Could you check a few things on this model? Use its own coordinates, in mm. A direction names the side the tool comes from. Coordinates: 2 decimals unless noted, no trailing zeros. Write each loop counter-clockwise with the first axis right and the second up, starting at its lowest first coordinate (ties: lowest second). Pieces come first, ordered by that corner, then holes. Notation, with made-up numbers: M -27,-25 L -2,-25 A4 ccw -2,-19 Z; hole C -21,49 d3. An arc over 180 degrees is marked long. Answer as CSV lines item,"result". Start each with the question number.
Item 1: Suppose I cut it at A-A, the plane x = -6. Write out the boundary of the cut face in (y, z), and give its area (3 significant figures).
Item 2: On a 3-axis mill with a long thin cutter (end or side, diameter ignored), from which of +Z, -Z, +X, -X, +Y, -Y can I reach the whole of each face in a straight line? I mean faces 3 (the cylindrical face through (35.965, 0.105, -27.525)), 4 (the flat face through (27.8, -2.5, -8)). Say none if no direction works.
Item 3: Suppose I cut it at C-C, the plane y = -1.25. Write out the boundary of the cut face in (x, z), and give its area (3 significant figures).
Item 4: If I drill on line 1 along Z through (x, y) = (-35.25, 0.5); line 2 along Z through (x, y) = (0, -6.1); line 3 along X through (y, z) = (-1, -14.5), over which ranges is the centre line in solid material (lowest first)? Write a range as [from, to].
Item 5: Suppose I cut it at B-B, the plane z = 0. Write out the boundary of the cut face in (x, y).
Item 6: We'd pull the mould along X, two halves only. Please class faces 1 (the flat face through (8, -7.5, 0)), 2 (the flat face through (35.5, 1, 0)): +X half, -X half, draft (parallel to the pull), parting line (faces both ways), or undercut.
Item 7: Suppose I cut it at D-D, the plane z = -12. Write out the boundary of the cut face in (x, y), and give its area (3 significant figures).
Item 8: I'm going to push flat-ended pins straight in: P1, Ø6, axis at x = -16, z = 23, coming from the +Y side; P2, Ø3.5, axis at x = 7.5, z = -22.5, coming from the +Y side; P3, Ø19.5, axis at x = 0, z = 0, coming from the -Y side; P4, Ø1.8, axis at x = -14, z = 0, coming from the +Y side. Where does each tip first touch, or does it pass through?
```python
from build123d import *

# Parameters (mm, degrees)
F0_W     = 75
F0_H     = 60
F0_R     = 0.75
F0_R_2   = 1.5
F0_R_3   = 7.5
F1_DEPTH = 7.5
F2_T     = -2
F3_DEPTH = 7.501
F4_R     = 1.5
F5_DEPTH = 3
F6_R     = 0.75
F7_DEPTH = 3


with BuildPart() as f1:
    # F0 (on Front) → F1 (new body, symmetric)
    with BuildSketch(Plane.XZ):
        Rectangle(F0_W, F0_H)
        with Locations((-35.25, -27.75)):
            Circle(F0_R, mode=Mode.SUBTRACT)
        with Locations((35.25, -27.75)):
            Circle(F0_R, mode=Mode.SUBTRACT)
        with Locations((-14, 0)):
            Circle(F0_R_2, mode=Mode.SUBTRACT)
        with Locations((-35.25, 27.75)):
            Circle(F0_R, mode=Mode.SUBTRACT)
        Circle(F0_R_3, mode=Mode.SUBTRACT)
        with Locations((14, 0)):
            Circle(F0_R_2, mode=Mode.SUBTRACT)
        with Locations((35.25, 27.75)):
            Circle(F0_R, mode=Mode.SUBTRACT)
        with Locations((-14, 0)):
            Circle(F0_R_2)
        Circle(F0_R_3)
        with Locations((14, 0)):
            Circle(F0_R_2)
    extrude(amount=F1_DEPTH, both=True)

    # F2
    f2_openings = [f1.faces().sort_by_distance(p)[0] for p in [
        (0, 7.5, 0),
    ]]
    offset(amount=F2_T, openings=f2_openings)

    # F0 (on Front) → F3 (cut, through all)
    with BuildSketch(Plane.XZ):
        with Locations((-14, 0)):
            Circle(F0_R_2)
        Circle(F0_R_3)
        with Locations((14, 0)):
            Circle(F0_R_2)
    extrude(amount=F3_DEPTH, mode=Mode.SUBTRACT)

    # F4 (on face) → F5 (join)
    with BuildSketch(Plane(origin=(0, -5.5, 0), x_dir=(-1, 0, 0), z_dir=(0, 1, 0))):
        with Locations((-28.4348707646, -7.3186149821)):
            Circle(F4_R)
        with Locations((-7.3929731734, -7.3186149821)):
            Circle(F4_R)
        with Locations((-28.4348707646, -23.2888292521)):
            Circle(F4_R)
        with Locations((-7.3929731734, -23.2888292521)):
            Circle(F4_R)
    extrude(amount=F5_DEPTH)

    # F6 (on face) → F7 (cut)
    with BuildSketch(Plane(origin=(0, -2.5, 0), x_dir=(-1, 0, 0), z_dir=(0, 1, 0))):
        with Locations((-28.4348707646, -7.3186149821)):
            Circle(F6_R)
    extrude(amount=-F7_DEPTH, mode=Mode.SUBTRACT)


solid = f1.part
```
Ans:
1,outline,"M -7.5,-30 L 7.5,-30 L 7.5,-28 L -5.5,-28 L -5.5,-4.5 L -7.5,-4.5 Z; M -7.5,4.5 L -5.5,4.5 L -5.5,28 L 7.5,28 L 7.5,30 L -7.5,30 Z"
1,area,"154 mm^2"
2,face 3,"+Y, -Y"
2,face 4,"+Y"
3,outline,"M -37.5,-30 L 37.5,-30 L 37.5,30 L -37.5,30 Z; hole C -35.25,-27.75 d1.5; hole C -35.25,27.75 d1.5; hole M -35.5,-25.01 A2.75 cw -32.51,-28 L 32.51,-28 A2.75 cw 35.5,-25.01 L 35.5,25.01 A2.75 cw 32.51,28 L -32.51,28 A2.75 cw -35.5,25.01 Z; hole C 35.25,-27.75 d1.5; hole C 35.25,27.75 d1.5"
3,area,"546 mm^2"
4,line 1,"z = [-30, -28.5], [-27, -25], [25, 27], [28.5, 30]"
4,line 2,"z = [-30, -7.5], [7.5, 30]"
4,line 3,"x = [-37.5, -35.5], [35.5, 37.5]"
5,outline,"M -37.5,-7.5 L -15.5,-7.5 L -15.5,-5.5 L -35.5,-5.5 L -35.5,7.5 L -37.5,7.5 Z; M -12.5,-7.5 L -7.5,-7.5 L -7.5,-5.5 L -12.5,-5.5 Z; M 7.5,-7.5 L 12.5,-7.5 L 12.5,-5.5 L 7.5,-5.5 Z; M 15.5,-7.5 L 37.5,-7.5 L 37.5,7.5 L 35.5,7.5 L 35.5,-5.5 L 15.5,-5.5 Z"
6,face 1,"draft"
6,face 2,"undercut"
7,outline,"M -37.5,-7.5 L 37.5,-7.5 L 37.5,7.5 L 35.5,7.5 L 35.5,-5.5 L -35.5,-5.5 L -35.5,7.5 L -37.5,7.5 Z"
7,area,"202 mm^2"
8,P1,"stops at y = -5.5"
8,P2,"stops at y = -2.5"
8,P3,"stops at y = -7.5"
8,P4,"passes through"
